from build123d import *

# Parameters (mm, degrees)
SKETCH_1_W                 = 120
SKETCH_1_H                 = 57
EXTRUDE_1_DEPTH            = 2
SKETCH_2_R                 = 1.6
CUT_EXTRUDE_1_DEPTH        = 67.454871906
CUT_EXTRUDE_2_DEPTH        = 67.454871906
PATTERN_LINEAR_1_COUNT     = 5
PATTERN_LINEAR_1_PITCH     = 12
PATTERN_LINEAR_1_COL_COUNT = 5
PATTERN_LINEAR_1_COL_PITCH = 12


with BuildPart() as part:
    # 草图1 → 凸台-拉伸1 (new body)
    with BuildSketch(Plane(origin=(0, 0, 0), x_dir=(1, 0, 0), z_dir=(0, 1, 0))):
        Rectangle(SKETCH_1_W, SKETCH_1_H)
    extrude(amount=EXTRUDE_1_DEPTH)

    # 草图2 → 切除-拉伸1 (cut, through all)
    with BuildSketch(Plane(origin=(0, 2, 0), x_dir=(1, 0, 0), z_dir=(0, 1, 0))):
        with Locations(Location((-57, 17.2, 0), (0, 0, 270))):
            Circle(SKETCH_2_R)
        with Locations(Location((-57, -2.8, 0), (0, 0, 270))):
            Circle(SKETCH_2_R)
        with Locations(Location((57, -2.8, 0), (0, 0, 90))):
            Circle(SKETCH_2_R)
        with Locations(Location((57, 17.2, 0), (0, 0, 90))):
            Circle(SKETCH_2_R)
    extrude(amount=-CUT_EXTRUDE_1_DEPTH, mode=Mode.SUBTRACT)

    # 草图3 → 切除-拉伸2 (cut, through all)
    with BuildSketch(Plane(origin=(0, 2, 0), x_dir=(1, 0, 0), z_dir=(0, 1, 0))):
        with BuildLine():
            ThreePointArc((-4, -18.5), (0, -14.5), (4, -18.5))
            Line((4, -18.5), (4, 18.5))
            ThreePointArc((4, 18.5), (0, 14.5), (-4, 18.5))
            Line((-4, 18.5), (-4, -18.5))
        make_face()
        with BuildLine():
            ThreePointArc((-4, 18.5), (0, 14.5), (4, 18.5))
            Line((4, 18.5), (-4, 18.5))
        make_face()
        with BuildLine():
            Line((-4, 18.5), (4, 18.5))
            ThreePointArc((4, 18.5), (0, 22.5), (-4, 18.5))
        make_face()
        with BuildLine():
            ThreePointArc((-4, -18.5), (0, -22.5), (4, -18.5))
            Line((4, -18.5), (-4, -18.5))
        make_face()
        with BuildLine():
            Line((-4, -18.5), (4, -18.5))
            ThreePointArc((4, -18.5), (0, -14.5), (-4, -18.5))
        make_face()
    cut_extrude_2 = extrude(amount=-CUT_EXTRUDE_2_DEPTH, mode=Mode.SUBTRACT)

    # 阵列(线性)1: 切除-拉伸2 ×5
    with Locations(*[(i * PATTERN_LINEAR_1_PITCH, 0, 0) for i in range(1, PATTERN_LINEAR_1_COUNT)]):
        add(cut_extrude_2, mode=Mode.SUBTRACT)

    # 阵列(线性)1 col: 切除-拉伸2 ×5
    with Locations(*[(-i * PATTERN_LINEAR_1_COL_PITCH, 0, 0) for i in range(1, PATTERN_LINEAR_1_COL_COUNT)]):
        add(cut_extrude_2, mode=Mode.SUBTRACT)


solid = part.part
Design review of the part built by this model. Coordinates are the model's own, in mm. Round coordinates to 2 decimals unless told otherwise and drop trailing zeros. Write each loop counter-clockwise with the first axis right and the second up, starting at its lowest first coordinate (ties: lowest second). Pieces come first, ordered by that corner, then holes. Notation, with made-up numbers: M 6.25,7.25 L 47.25,7.25 A12 ccw 47.25,29.25 Z; hole C -35.75,-12.5 d2. An arc over 180 degrees is marked long. One line per item, written item: value. Start each with the question number.
1. To check wall thickness, follow probe 1 along Z at (x, y) = (57, 0.55); probe 2 along Z at (x, y) = (-9, 1.55); probe 3 along Z at (x, y) = (39.5, 1.2). State the ranges of each line that lie inside material, in increasing order. Write a range as from..to.
2. Take a section at B-B on y = 1. State how many separate pieces and enclosed holes the cut face has, then the cut area to 3 significant figures.
3. Draft analysis for pull direction Z (two halves, no side actions). For faces 1 (the face through (-55.65, 1.01, 3.66)), 2 (the face through (-14, 0, 25)), state which applies: pulls with the +Z half, pulls with the -Z half, needs draft (parallel to the pull), parting line crosses it, or undercut.
4. Take a section at A-A on x = 24. State the section outline as (y, z) points.
5. Take a section at D-D on x = -1. State the section outline as (y, z) points, then the cut area to 3 significant figures.
Computed:
1. probe 1: z = -28.5..-18.8, -15.6..1.2, 4.4..28.5
1. probe 2: z = -28.5..-21.15, 21.15..28.5
1. probe 3: z = -28.5..-20.44, 20.44..28.5
2. separate pieces: 1
2. enclosed holes: 13
2. area: 3,690 mm²
3. face 1: undercut
3. face 2: needs draft
4. outline: M 0,-28.5 L 2,-28.5 L 2,-22.5 L 0,-22.5 Z; M 0,22.5 L 2,22.5 L 2,28.5 L 0,28.5 Z
5. outline: M 0,-28.5 L 2,-28.5 L 2,-22.37 L 0,-22.37 Z; M 0,22.37 L 2,22.37 L 2,28.5 L 0,28.5 Z
5. area: 24.5 mm²
